```python
from build123d import *

# Parameters (mm, degrees)
SKETCH1_W                               = 50
SKETCH1_H                               = 80
BOSS_EXTRUDE1_DEPTH                     = 5
BOSS_EXTRUDE2_DEPTH                     = 10
SKETCH1_4_W                             = 4
SKETCH1_4_H                             = 80
BOSS_EXTRUDE3_DEPTH                     = 30
CBORE_FOR_M5_HEX_HEAD_BOLT1_D           = 3
CBORE_FOR_M5_HEX_HEAD_BOLT1_CBORE_D     = 5.7
CBORE_FOR_M5_HEX_HEAD_BOLT1_CBORE_DEPTH = 3.2


with BuildPart() as part:
    # Sketch1 → Boss-Extrude1 (new body)
    with BuildSketch(Plane(origin=(0, 0, 0), x_dir=(1, 0, 0), z_dir=(0, 1, 0))):
        with Locations((-26.495327103, -4.236760125)):
            Rectangle(SKETCH1_W, SKETCH1_H)
    extrude(amount=BOSS_EXTRUDE1_DEPTH)

    # Sketch1<3> → Boss-Extrude2 (add)
    with BuildSketch(Plane(origin=(0, 0, 0), x_dir=(1, 0, 0), z_dir=(0, 1, 0))):
        Polygon((-55.495327103, 35.763239875), (-51.495327103, 35.763239875), (-1.495327103, 35.763239875), (-1.495327103, 39.763239875), (-55.495327103, 39.763239875), align=None)
    extrude(amount=BOSS_EXTRUDE2_DEPTH)

    # Sketch1<4> → Boss-Extrude3 (add)
    with BuildSketch(Plane(origin=(0, 0, 0), x_dir=(1, 0, 0), z_dir=(0, 1, 0))):
        with Locations((-53.495327103, -4.236760125)):
            Rectangle(SKETCH1_4_W, SKETCH1_4_H)
    extrude(amount=BOSS_EXTRUDE3_DEPTH)

    # CBORE for M5 Hex Head Bolt1 (through all)
    with Locations(Plane(origin=(-25.6653615, 5, -85), x_dir=(1, 0, 0), z_dir=(0, 1, 0))):
        with Locations((-0.829965603, -69.236760125), (-0.829965603, -109.236760125)):
            CounterBoreHole(CBORE_FOR_M5_HEX_HEAD_BOLT1_D / 2, CBORE_FOR_M5_HEX_HEAD_BOLT1_CBORE_D / 2, CBORE_FOR_M5_HEX_HEAD_BOLT1_CBORE_DEPTH)


solid = part.part
```
CAD build for the part. Positions are in the model's coordinates, mm. A direction names the side the tool comes from. Give positions to 0.01 mm unless a question says otherwise; leave off trailing zeros. Order: outer loops, then holes, each group sorted by start corner. A loop starts at its lowest first (then second) coordinate and runs counter-clockwise, first axis right, second up.
(1) Drill centre lines: L1, parallel to Z at x = -13, y = 8.5; L2, parallel to X at y = 11, z = 40.5; L3, parallel to Y at x = -49.5, z = -4. Where is each one in solid material? Low to high.
(2) Flat gauge pins, fed straight in: pin 1 (3 mm diameter, centred on x = -18, z = -38, fed in from +Y); pin 2 (6.5 mm diameter, centred on x = -25.5, z = -15.5, fed in from +Y); pin 3 (3 mm diameter, centred on x = -27.5, z = 25, fed in from +Y). Where does each tip first touch, or does it go through?
(3) Saw through at C-C, the plane z = 5.5. Give the cut face in (x, y).
(4) Mould opens along X. For faces 5 (the flat face through (-1.495, 3, 3)), 6 (the flat face through (-27, 7, -35.763)), 7 (the cylindrical face through (-23.863, 3.422, -14.672)), 8 (the flat face through (-55.495, 15, 3)) say: released by +X, released by -X, zero draft, split by the parting line, or undercut.
(5) Saw through at B-B, the plane y = 6. Give the cut face in (x, z), then the cut area to 3 significant figures.
(6) Saw through at A-A, the plane x = -26.5. Give the cut face in (y, z), then the cut area to 3 significant figures.
(7) Saw through at D-D, the plane y = 13.5. Give the cut face in (x, z).
(8) Tool access for faces 1 (the flat face through (-27, 5, 4)), 2 (the flat face through (-54, 30, 4)), 3 (the flat face through (-54, 20, -35.763)), 4 (the flat face through (-25, 1.8, 25)): list every direction of +Z, -Z, +X, -X, +Y, -Y with a clear straight run to the whole face (end or side of a thin tool).
Results found:
1. L1: z = -39.76 to -35.76
1. L2: x = -55.5 to -51.5
1. L3: y = 0 to 5
2. pin 1: stops at y = 10
2. pin 2: stops at y = 5
2. pin 3: stops at y = 1.8
3. outline: (-55.5, 0) - (-1.5, 0) - (-1.5, 5) - (-51.5, 5) - (-51.5, 30) - (-55.5, 30) - close
4. face 5: released by +X
4. face 6: zero draft
4. face 7: undercut
4. face 8: released by -X
5. outline: (-55.5, -39.76) - (-1.5, -39.76) - (-1.5, -35.76) - (-51.5, -35.76) - (-51.5, 44.24) - (-55.5, 44.24) - close
5. area: 536 mm2
6. outline: (0, -39.76) - (10, -39.76) - (10, -35.76) - (5, -35.76) - (5, -18.61) - (1.8, -18.61) - (1.8, -17.26) - (0, -17.26) - close; (0, -14.26) - (1.8, -14.26) - (1.8, -12.91) - (5, -12.91) - (5, 21.39) - (1.8, 21.39) - (1.8, 22.74) - (0, 22.74) - close; (0, 25.74) - (1.8, 25.74) - (1.8, 27.09) - (5, 27.09) - (5, 44.24) - (0, 44.24) - close
6. area: 393 mm2
7. outline: (-55.5, -35.76) - (-51.5, -35.76) - (-51.5, 44.24) - (-55.5, 44.24) - close
8. face 1: +Z, +X, +Y
8. face 2: +Z, -Z, +X, -X, +Y
8. face 3: -Z, +X, -X, +Y
8. face 4: +Y
